from build123d import *

# Parameters (mm, degrees)
SKETCH_1_R          = 5
EXTRUDE_1_DEPTH     = 2
EXTRUDE_2_DEPTH     = 3.5
EXTRUDE_3_DEPTH     = 3.5
SKETCH_4_R          = 5
EXTRUDE_4_DEPTH     = 0.5
CUT_EXTRUDE_2_DEPTH = 3
CUT_EXTRUDE_3_DEPTH = 2
EXTRUDE_5_DEPTH     = 58
SKETCH_8_R          = 5
EXTRUDE_6_DEPTH     = 58
CUT_EXTRUDE_4_DEPTH = 8
SKETCH_10_R         = 1.5
CUT_EXTRUDE_5_DEPTH = 15
SKETCH_11_R         = 3.5
CUT_EXTRUDE_6_DEPTH = 30
SKETCH_12_R         = 1
CUT_EXTRUDE_7_DEPTH = 7
SKETCH_13_R         = 3.5
SKETCH_14_R         = 1


# Read off the part's stored shape, not the designer's step: 切除-扫描1
with BuildPart() as part:
    # 草图1 → 凸台-拉伸1 (new body)
    with BuildSketch(Plane(origin=(0, 0, 0), x_dir=(1, 0, 0), z_dir=(0, 1, 0))):
        with Locations(Location((0, 0, 0), (0, 0, 270))):
            Circle(SKETCH_1_R)
        Polygon((2.55392077, -1.838021228), (2.868733461, 1.292749652), (0.314812691, 3.13077088), (-2.55392077, 1.838021228), (-2.868733461, -1.292749652), (-0.314812691, -3.13077088), align=None, mode=Mode.SUBTRACT)
    extrude(amount=EXTRUDE_1_DEPTH)

    # 草图2 → 凸台-拉伸2 (add)
    with BuildSketch(Plane(origin=(0, 2, 0), x_dir=(1, 0, 0), z_dir=(0, 1, 0))):
        Polygon((-2.834872538, 1.792623133), (3.135022029, 1.192324151), (2.834872538, -1.792623133), (-3.135022029, -1.192324151), align=None)
    extrude(amount=EXTRUDE_2_DEPTH)

    # 草图3 → 凸台-拉伸3 (add)
    with BuildSketch(Plane(origin=(0, 2, 0), x_dir=(1, 0, 0), z_dir=(0, 1, 0))):
        Polygon((-1.192324151, 3.135022029), (-1.792623133, -2.834872538), (1.192324151, -3.135022029), (1.792623133, 2.834872538), align=None)
    extrude(amount=EXTRUDE_3_DEPTH)

    # 草图4 → 凸台-拉伸4 (add)
    with BuildSketch(Plane(origin=(0, 2, 0), x_dir=(1, 0, 0), z_dir=(0, 1, 0))):
        with Locations(Location((0, 0, 0), (0, 0, 270))):
            Circle(SKETCH_4_R)
    extrude(amount=EXTRUDE_4_DEPTH)

    # 草图5 → 切除-拉伸2 (cut)
    with BuildSketch(Plane(origin=(0, 5.5, 0), x_dir=(1, 0, 0), z_dir=(0, 1, 0))):
        Polygon((-3.135022029, -1.192324151), (-2.834872538, 1.792623133), (-1.342398896, 1.642548387), (-1.192324151, 3.135022029), (1.792623133, 2.834872538), (1.642548387, 1.342398896), (3.135022029, 1.192324151), (2.834872538, -1.792623133), (1.342398896, -1.642548387), (1.192324151, -3.135022029), (-1.792623133, -2.834872538), (-1.642548387, -1.342398896), align=None)
        Polygon((-1.093653289, 1.617535929), (-0.968591001, 2.861263964), (1.518865068, 2.611139388), (1.39380278, 1.367411354), (1.368790323, 1.118665747), (1.617535929, 1.093653289), (2.861263964, 0.968591001), (2.611139388, -1.518865068), (1.367411354, -1.39380278), (1.118665747, -1.368790323), (1.093653289, -1.617535929), (0.968591001, -2.861263964), (-1.518865068, -2.611139388), (-1.39380278, -1.367411354), (-1.368790323, -1.118665747), (-1.617535929, -1.093653289), (-2.861263964, -0.968591001), (-2.611139388, 1.518865068), (-1.367411354, 1.39380278), (-1.118665747, 1.368790323), align=None, mode=Mode.SUBTRACT)
    extrude(amount=-CUT_EXTRUDE_2_DEPTH, mode=Mode.SUBTRACT)

    # 草图6 → 切除-拉伸3 (cut)
    with BuildSketch(Plane.XZ):
        Polygon((2.888759724, -1.318484202), (2.586220675, 1.842497205), (-0.302539048, 3.160981407), (-2.888759724, 1.318484202), (-2.586220675, -1.842497205), (0.302539048, -3.160981407), align=None)
    extrude(amount=-CUT_EXTRUDE_3_DEPTH, mode=Mode.SUBTRACT)

    # 草图7 → 凸台-拉伸5 (add)
    with BuildSketch(Plane(origin=(0, 5.5, 0), x_dir=(1, 0, 0), z_dir=(0, 1, 0))):
        Polygon((-1.118665747, 1.368790323), (-0.968591001, 2.861263964), (1.518865068, 2.611139388), (1.368790323, 1.118665747), (2.861263964, 0.968591001), (2.611139388, -1.518865068), (1.118665747, -1.368790323), (0.968591001, -2.861263964), (-1.518865068, -2.611139388), (-1.368790323, -1.118665747), (-2.861263964, -0.968591001), (-2.611139388, 1.518865068), align=None)
    extrude(amount=EXTRUDE_5_DEPTH)

    # 草图8 → 凸台-拉伸6 (add)
    with BuildSketch(Plane(origin=(0, 2.5, 0), x_dir=(1, 0, 0), z_dir=(0, 1, 0))):
        with Locations(Location((0, 0, 0), (0, 0, 270))):
            Circle(SKETCH_8_R)
    extrude(amount=EXTRUDE_6_DEPTH)

    # 草图9 → 切除-拉伸4 (cut)
    with BuildSketch(Plane.XZ):
        Polygon((2.888759724, -1.318484202), (2.586220675, 1.842497205), (-0.302539048, 3.160981407), (-2.888759724, 1.318484202), (-2.586220675, -1.842497205), (0.302539048, -3.160981407), align=None)
    extrude(amount=-CUT_EXTRUDE_4_DEPTH, mode=Mode.SUBTRACT)

    # 草图10 → 切除-拉伸5 (cut)
    with BuildSketch(Plane.XZ.offset(-8)):
        with Locations(Location((0, 0, 0), (0, 0, 270))):
            Circle(SKETCH_10_R)
    extrude(amount=-CUT_EXTRUDE_5_DEPTH, mode=Mode.SUBTRACT)

    # 草图11 → 切除-拉伸6 (cut)
    with BuildSketch(Plane.XZ.offset(-23)):
        with Locations(Location((0, 0, 0), (0, 0, 270))):
            Circle(SKETCH_11_R)
    extrude(amount=-CUT_EXTRUDE_6_DEPTH, mode=Mode.SUBTRACT)

    # 草图12 → 切除-拉伸7 (cut)
    with BuildSketch(Plane.XZ.offset(-53)):
        with Locations(Location((0, 0, 0), (0, 0, 270))):
            Circle(SKETCH_12_R)
    extrude(amount=-CUT_EXTRUDE_7_DEPTH, mode=Mode.SUBTRACT)

    # 草图13 → 放样1 section 0
    with BuildSketch(Plane.XZ.offset(-53)):
        Circle(SKETCH_13_R)
    # 草图14 → 放样1 section 1
    with BuildSketch(Plane.XZ.offset(-60)):
        Circle(SKETCH_14_R)
    loft()

    # 切除-扫描1 outline → 切除-扫描1 (revolve, cut)
    with BuildSketch(Plane.XY):
        Polygon((3.5, 53), (0, 60.5), (0, 53), align=None)
    revolve(axis=Axis((0, 0, 0), (0, 1, 0)), mode=Mode.SUBTRACT)


solid = part.part
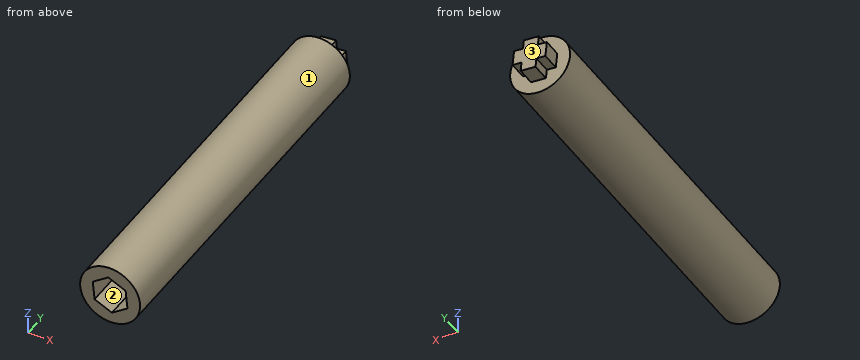
Can you work these out from the model? Positions are in its coordinate system, mm. Face numbers are marked on the shaded views. Coordinates: 2 decimals unless noted, no trailing zeros. Order: outer loops, then holes, each group sorted by start corner. A loop starts at its lowest first (then second) coordinate and runs counter-clockwise, first axis right, second up. Notation, with made-up numbers: (52.5, 1) - (62.5, 1) arc R25 cw to (62.5, 21) - close; hole circle Ø4 at (13, 7.25). An arc over 180 degrees is marked (long way). Answer as a JSON object with one key per item and string values. Group by question number.
Q1. We'd pull the mould along X, two halves only. Please class the marked faces 1, 2 and 3: +X half, -X half, draft (parallel to the pull), parting line (faces both ways), or undercut.
Q2. Imagine slicing it at A-A (y = 6). Please give me the cut outline in (x, z).
Q3. Will these pins go through, and if not, where does the flat tip stop? P1, Ø4, axis at x = -0.5, y = 42.5, coming from the +Z side; P2, Ø2, axis at x = 4, y = 43.5, coming from the +Z side; P3, Ø1.8, axis at x = 0, z = 0, coming from the -Y side; P4, Ø1.5, axis at x = 1, y = 14.5, coming from the -Z side.
Q4. I need wall thicknesses on line 1 (X direction, y = 32.5, z = 0); line 2 (X direction, y = 14.5, z = 0); line 3 (Y direction, x = -3.75, z = -3). Which ranges of each line are inside material? Lowest first, please. Write a range as from..to.
Q5. Imagine slicing it at B-B (y = 45). Please give me the cut outline in (x, z), and give its area (3 significant figures).
Determined:
{
 "1": {"face 1": "parting line", "face 2": "undercut", "face 3": "draft"},
 "2": {"outline": "circle Ø10 at (0, 0); hole (-2.89, 1.32) - (-2.59, -1.84) - (0.3, -3.16) - (2.89, -1.32) - (2.59, 1.84) - (-0.3, 3.16) - close"},
 "3": {"P1": "stops at z = 5", "P2": "stops at z = 4", "P3": "stops at y = 58.57", "P4": "stops at z = -4.99"},
 "4": {"line 1": "x = -5..-3.5, 3.5..5", "line 2": "x = -5..-1.5, 1.5..5", "line 3": "y = 0..60.5"},
 "5": {"outline": "circle Ø10 at (0, 0); hole circle Ø7 at (0, 0)", "area": "40.1 mm2"}
}
